Autodesk Inventor part; units mm, degrees
ref_plane "YZ Plane" through (0, 0, 0) normal (1, 0, 0) x (0, 1, 0)
ref_plane "XZ Plane" through (0, 0, 0) normal (0, 1, 0) x (-1, 0, 0)
ref_plane "XY Plane" through (0, 0, 0) normal (0, 0, 1) x (1, 0, 0)
sketch "Sketch1" plane through (0, 0, 0) normal (0, 1, 0) x (-1, 0, 0)
  line L0 (0, 0) -> (-2.54, 0)
  line L1 (-2.54, 0) -> (-2.54, -12.7)
  line L2 (-2.54, -12.7) -> (0, -12.7)
  line L3 (0, -12.7) -> (0, 0)
  line L4 (0, -12.7) -> (-12.7, -12.7)
  line L5 (-12.7, -12.7) -> (-12.7, -10.16)
  line L6 (-12.7, -10.16) -> (0, -10.16)
  line L7 (0, -10.16) -> (0, -12.7)
  dimension "d0" = 12.7
  dimension "d1" = 12.7
  dimension "d2" = 2.54
  dimension "d3" = 2.54
extrude "Extrusion1" add sketch "Sketch1" along normal blind 50.8
sketch "Sketch2" plane through (0, 50.8, 0) normal (0, 1, 0) x (1, 0, 0)
  line L0 (2.54, 0) -> (-7.62, 0)
  line L1 (-7.62, 0) -> (-7.62, 20.32)
  line L2 (-7.62, 20.32) -> (2.54, 20.32)
  line L3 (2.54, 20.32) -> (2.54, 0)
  line L4 (12.7, 10.16) -> (12.7, 12.7)
  line L5 (12.7, 10.16) -> (-7.62, 10.16)
  line L6 (-7.62, 10.16) -> (-7.62, 20.32)
  line L7 (-7.62, 20.32) -> (12.7, 20.32)
  line L8 (12.7, 20.32) -> (12.7, 10.16)
  line L9 (2.54, 0) -> (2.54, 10.16)
  point P0 (0, 0)
  dimension "d6" = 10.16
  dimension "d7" = 0
  dimension "d8" = 10.16
  dimension "d9" = 20.32
extrude "Extrusion2" add sketch "Sketch2" along normal blind 6.35
sketch "Sketch3" plane through (0, 50.8, 0) normal (0, -1, 0) x (1, 0, 0)
  line L0 (-7.62, -20.32) -> (12.7, -20.32)
  line L1 (12.7, -20.32) -> (-7.62, -20.32)
  line L2 (-7.62, -20.32) -> (-7.62, -16.383)
  line L3 (-7.62, -16.383) -> (12.7, -16.383)
  line L4 (12.7, -16.383) -> (12.7, -20.32)
  line L5 (-7.62, 0) -> (-3.683, 0)
  line L6 (-3.683, 0) -> (-3.683, -20.32)
  line L7 (-3.683, -20.32) -> (-7.62, -20.32)
  line L8 (-7.62, -20.32) -> (-7.62, 0)
  line L9 (0, -12.7) -> (0, 0)
  line L10 (12.7, -12.7) -> (0, -12.7)
  dimension "d12" = 3.683
  dimension "d13" = 3.683
extrude "Extrusion3" add sketch "Sketch3" along normal blind 12.7
sketch "Sketch4" plane through (-7.62, 57.15, -20.32) normal (-1, 0, 0) x (0, 0, 1)
  line L0 (20.32, 0) -> (20.32, -19.05)
  line L1 (0, 0) -> (20.32, 0)
  point P0 (20.32, -57.15)
  point P1 (16.51, -12.7)
  point P2 (20.32, -6.35)
  dimension "d16" = 3.81
  dimension "d27" = 6.35
hole "Hole1" at (-7.62, 44.45, -3.81) direction (1, 0, 0) diameter 3.81 depth 4.318 tip angle 118
sketch "Sketch5" plane through (12.7, 57.15, -20.32) normal (0, 0, -1) x (-1, 0, 0)
  line L0 (16.383, -6.35) -> (0, -6.35)
  line L1 (0, 0) -> (0, -19.05)
  point P0 (12.7, -57.15)
  point P1 (3.81, -12.7)
  dimension "d28" = 6.35
  dimension "d29" = 3.81
hole "Hole2" at (8.89, 44.45, -20.32) direction (0, 0, 1) diameter 3.81 depth 4.445 tip angle 118
sketch "Sketch6" plane through (0, 0, 0) normal (0, 1, 0) x (-1, 0, 0)
  line L0 (-2.54, 0) -> (-2.54, -10.16)
  line L1 (-2.54, 0) -> (-5.334, 0)
  line L2 (-5.334, 0) -> (-5.334, -10.16)
  line L3 (-5.334, -10.16) -> (-2.54, -10.16)
  line L4 (-2.54, -10.16) -> (-2.54, 0)
  line L5 (-2.54, -10.16) -> (-12.7, -10.16)
  line L6 (-12.7, -10.16) -> (-2.54, -10.16)
  line L7 (-2.54, -10.16) -> (-2.54, -7.366)
  line L8 (-2.54, -7.366) -> (-12.7, -7.366)
  line L9 (-12.7, -7.366) -> (-12.7, -10.16)
  point P0 (0, 0)
  dimension "d37" = 2.794
  dimension "d38" = 2.794
extrude "Extrusion4" add sketch "Sketch6" along normal blind 57.15
equation "\"d38\" = d37"
properties part number "TelescopeGroot 8"
Input: part model. Units: mm. Frame: model coordinates. A direction names the side the tool comes from. Coordinates: 2 decimals unless noted, no trailing zeros. Loops run counter-clockwise (first coordinate to the right, second up) from the corner with the lowest first, then second, coordinate; pieces in that order, holes last. Notation, with made-up numbers: M 1.25,16 L 6.25,16 A26 cw 6.25,54 Z; hole C 83.25,39.5 d5. An arc over 180 degrees is marked long. Use a Markdown table: item, result. Add a question column.
1) Section D-D, the plane x = 4. Return the cut outline in (y, z), plus the area to 3 significant figures.
2) Line query: L1, parallel to Y at x = 8.89, z = -18.35 (3 decimals); L2, parallel to Z at x = -5.5, y = 44.45 (3 decimals); L3, parallel to Y at x = -2.5, z = -15.75. Output: solid intervals per line, ascending. Write a range as from..to.
3) Section B-B, the plane x = 8.89. Return the cut outline in (y, z) (3 decimals), plus the area to 3 significant figures.
4) Pin query (flat end, axial travel): P1, Ø2, axis at y = 25.5, z = -2.5, coming from the -X side; P2, Ø6.5, axis at x = 4.5, y = 17, coming from the -Z side; P3, Ø3.5, axis at y = 44.45, z = -3.81, coming from the +X side. Return the tip coordinate at first contact, or that it passes through.
5) Set-up query: faces 1 (the flat face through (-4, 38.1, -15)), 2 (the flat face through (6, 25, -12.7)), 3 (the flat face through (-3.683, 45, -8)). Return all of +Z, -Z, +X, -X, +Y, -Y with unobstructed straight access to the full face (end or side cutting, diameter ignored); none if empty.
6) Section A-A, the plane z = -3.81. Return the cut outline in (x, y) (3 decimals), plus the area to 3 significant figures.
7) Section C-C, the plane y = 44.45. Return the cut outline in (x, z) (3 decimals).
8) Draft query along Z for faces 4 (the flat face through (9, 28, -7.366)), 5 (the flat face through (4, 45, -16.383)), 6 (the flat face through (5.334, 28, -4)), 7 (the cylindrical face through (-5.62, 46.31, -4.22)). Return one class per face: +Z half, -Z half, draft (parallel to the pull), parting line (faces both ways), or undercut.
Answer below:
| question | item | result |
|---|---|---|
| 1 | outline | M 0,-12.7 L 50.8,-12.7 L 50.8,-16.38 L 38.1,-16.38 L 38.1,-20.32 L 57.15,-20.32 L 57.15,0 L 0,0 Z |
| 1 | area | 824 mm2 |
| 2 | L1 | 38.1..42.545, 46.355..57.15 |
| 2 | L2 | -20.32..-5.715, -1.905..0 |
| 2 | L3 | 50.8..57.15 |
| 3 | outline | M 0,-12.7 L 50.8,-12.7 L 50.8,-16.383 L 46.355,-16.383 L 46.355,-20.32 L 57.15,-20.32 L 57.15,-7.366 L 0,-7.366 Z; M 38.1,-20.32 L 42.545,-20.32 L 42.545,-16.383 L 38.1,-16.383 Z |
| 3 | area | 388 mm2 |
| 4 | P1 | x = 0 |
| 4 | P2 | z = -12.7 |
| 4 | P3 | x = 5.33 |
| 5 | face 1 | -Z, -X, -Y |
| 5 | face 2 | +X, -Y |
| 5 | face 3 | +Z, -Y |
| 6 | outline | M -7.62,38.1 L -3.683,38.1 L -3.683,42.545 L -7.62,42.545 Z; M -7.62,46.355 L -3.683,46.355 L -3.683,50.8 L 0,50.8 L 0,0 L 5.334,0 L 5.334,57.15 L -7.62,57.15 Z |
| 6 | area | 388 mm2 |
| 7 | outline | M -7.62,-20.32 L 6.985,-20.32 L 6.985,-16.383 L -3.683,-16.383 L -3.683,-5.715 L -7.62,-5.715 Z; M -7.62,-1.905 L -3.683,-1.905 L -3.683,0 L -7.62,0 Z; M 0,-12.7 L 12.7,-12.7 L 12.7,-7.366 L 5.334,-7.366 L 5.334,0 L 0,0 Z; M 10.795,-20.32 L 12.7,-20.32 L 12.7,-16.383 L 10.795,-16.383 Z |
| 8 | face 4 | +Z half |
| 8 | face 5 | undercut |
| 8 | face 6 | draft |
| 8 | face 7 | undercut |
